```python
from build123d import *

# Parameters (mm, degrees)
F0_R            = 40.8
F1_DEPTH        = 8
F4_R            = 3.15
F6_W            = 4.8
F6_H            = 38.4
F7_DEPTH        = 8.001
F9_DEPTH        = 8
F10_R           = 21
F11_DEPTH       = 8.001
F12_R           = 4
F14_D           = 3.3
F14_CBORE_D     = 6.5
F14_CBORE_DEPTH = 3
F15_SIZE        = 0.5


with BuildPart() as f1:
    # F0 (on Top) → F1 (new body)
    with BuildSketch(Plane.XY):
        Circle(F0_R)
    extrude(amount=F1_DEPTH)

    # F2 (on Right) → F3 (revolve, cut)
    with BuildSketch(Plane.YZ):
        Polygon((0, 8), (0, 0), (8.6, 0), (8.6, 6), (6.5, 6), (6.5, 8), align=None)
    revolve(axis=Axis((0, 0, 10.7360328796), (0, 0, 1)), mode=Mode.SUBTRACT)

    # F4 (on Right) → F5 (revolve, cut)
    with BuildSketch(Plane.YZ):
        with Locations((31, 9)):
            Circle(F4_R)
    revolve(axis=Axis((0, 0, 6.3867427816), (0, 0, 1)), mode=Mode.SUBTRACT)

    # F6 (on Top) → F7 (cut, through all)
    with BuildSketch(Plane.XY):
        with Locations((-38.4, 0)):
            Rectangle(F6_W, F6_H)
    extrude(amount=F7_DEPTH, mode=Mode.SUBTRACT)

    # F8 (on Top) → F9 (join, through all)
    with BuildSketch(Plane.XY):
        with BuildLine():
            Line((-45, 28.2782724184), (-45, -28.2782724184))
            Line((-45, -28.2782724184), (-12.6078933705, -38.8031058648))
            ThreePointArc((-12.6078933705, -38.8031058648), (-26.2059585661, -31.2711965814), (-36, -19.2))
            Line((-36, -19.2), (-36, 19.2))
            ThreePointArc((-36, 19.2), (-26.2059585661, 31.2711965814), (-12.6078933705, 38.8031058648))
            Line((-12.6078933705, 38.8031058648), (-45, 28.2782724184))
        make_face()
    extrude(amount=F9_DEPTH)

    # F10 (on face) → F11 (cut, through all)
    with BuildSketch(Plane.XY.offset(8)):
        with Locations((-56.25, 0)):
            Circle(F10_R)
    extrude(amount=-F11_DEPTH, mode=Mode.SUBTRACT)

    # F12
    f12_edges = [f1.edges().sort_by_distance(p)[0] for p in [
        (-45, -17.732386, 4),
        (-45, 17.732386, 4),
    ]]
    fillet(f12_edges, radius=F12_R)

    # F14 (through all)
    with Locations(Plane.XY.offset(8)):
        with Locations((-40.5, 24), (-40.5, -24), (37.5, 0)):
            CounterBoreHole(F14_D / 2, F14_CBORE_D / 2, F14_CBORE_DEPTH)

    # F15
    f15_edges = [f1.edges().sort_by_distance(p)[0] for p in [
        (-45, 24.044154, 0),
        (-44.588872, 18.043683, 0),
        (-28.803947, 33.540689, 0),
        (-35.25, 0, 0),
        (40.8, 0, 0),
        (-44.588872, -18.043683, 0),
        (-28.803947, -33.540689, 0),
        (-45, -24.044154, 0),
        (-42.15, -24, 0),
        (-42.15, 24, 0),
        (0, -8.6, 0),
        (35.85, 0, 0),
    ]]
    chamfer(f15_edges, length=F15_SIZE)


solid = f1.part
```
Work out the finished part from the listing and answer in its coordinate system (mm). A direction names the side the tool comes from. Coordinates: 2 decimals unless noted, no trailing zeros. Write each loop counter-clockwise with the first axis right and the second up, starting at its lowest first coordinate (ties: lowest second). Pieces come first, ordered by that corner, then holes. Notation, with made-up numbers: (23, 75.5) - (80, 75.5) arc R29 cw to (80, 103.5) - close; hole circle Ø1 at (29.25, -27). An arc over 180 degrees is marked (long way). Answer as a JSON object with one key per item and string values.
Q1. Find section A-A (y = 0). State how many separate pieces and enclosed holes the cut face has, plus the area to 3 significant figures.
Results list:
{"separate pieces": "3", "enclosed holes": "0", "area": "424 mm^2"}
Q2. For a pull along Y with two mould halves and no side action, classify faces 1 (the cylindrical face through (39.15, 0.07, 2.72)), 2 (the cylindrical face through (40.786, -1.077, 4.198)), 3 (the flat face through (-7, 0, 8)), 4 (the flat face through (-28.95, -33.23, 0.25)) as pulls with the +Y half, pulls with the -Y half, needs draft (parallel to the pull), parting line crosses it, or undercut.
Results list:
{"face 1": "undercut", "face 2": "parting line crosses it", "face 3": "needs draft", "face 4": "pulls with the -Y half"}
Q3. Find section B-B (z = 2.75). Write down the section's boundary in (x, y), plus the area to 3 significant figures.
Results list:
{"outline": "(-45, -28.28) - (-12.61, -38.8) arc R40.8 ccw (long way) to (-12.61, 38.8) - (-45, 28.28) - (-45, 19.81) arc R4 ccw to (-43.44, 16.64) arc R21 cw to (-43.44, -16.64) arc R4 ccw to (-45, -19.81) - close; hole circle Ø3.3 at (-40.5, -24); hole circle Ø3.3 at (-40.5, 24); hole circle Ø17.2 at (0, 0); hole circle Ø3.3 at (37.5, 0)", "area": "5,300 mm^2"}
Q4. Consider L1, parallel to Y at x = 0, z = 6.4; L2, parallel to Y at x = 0, z = 2.75; L3, parallel to Y at x = -40.5, z = 3.2. Determine where each line is inside the solid, lowest interval first. Write a range as from..to.
Results list:
{"L1": "y = -40.8..-32.78, -29.22..-6.5, 6.5..29.22, 32.78..40.8", "L2": "y = -40.8..-8.6, 8.6..40.8", "L3": "y = -29.74..-25.65, -22.35..-13.89, 13.89..22.35, 25.65..29.74"}
Q5. Which of the six approach directions +Z, -Z, +X, -X, +Y, -Y give full straight-line access (tool end or side, diameter ignored) to faces 5 (the flat face through (-42, 25, 5)), 6 (the cylindrical face through (-39.284, 25.115, 2.719)), 7 (the flat face through (-29.031, -33.467, 4.198)), 8 (the flat face through (-6, -3, 6)), 9 (the cylindrical face through (-44.6, -18.07, 4.3))?
Results list:
{"face 5": "+Z", "face 6": "+Z, -Z", "face 7": "+Z, -Z, -X, -Y", "face 8": "-Z", "face 9": "+Z, -Z, -X"}
Q6. Given pin 1 Ø14 at (x, y) = (0, 0) entering from -Z; pin 2 Ø19 at (x, y) = (-1, 0.5) entering from -Z; pin 3 Ø2 at (x, z) = (-20.5, 4) entering from -Y; pin 4 Ø2 at (x, y) = (-39, -24.5) entering from +Z, each flat-ended and moving along its own axis, determine where each tip first touches the part or whether it passes through.
Results list:
{"pin 1": "stops at z = 6", "pin 2": "stops at z = 0", "pin 3": "stops at y = -36.56", "pin 4": "stops at z = 5"}
Q7. Find section C-C (x = 0). Write down the section's boundary in (y, z), plus the area to 3 significant figures.
Results list:
{"outline": "(-40.8, 0.5) - (-40.3, 0) - (-9.1, 0) - (-8.6, 0.5) - (-8.6, 6) - (-6.5, 6) - (-6.5, 8) - (-28.01, 8) arc R3.15 cw to (-33.99, 8) - (-40.8, 8) - close; (6.5, 6) - (8.6, 6) - (8.6, 0.5) - (9.1, 0) - (40.3, 0) - (40.8, 0.5) - (40.8, 8) - (33.99, 8) arc R3.15 cw to (28.01, 8) - (6.5, 8) - close", "area": "504 mm^2"}
